from build123d import *

# Parameters (mm, degrees)
SKETCH1_W           = 30
SKETCH1_H           = 50
BOSS_EXTRUDE1_DEPTH = 10
SHELL1_T            = -3
CUT_EXTRUDE1_REACH  = 32.822
SKETCH2_R           = 1.5
SKETCH2_R_2         = 2.75
CUT_EXTRUDE2_REACH  = 42.311
SKETCH3_W           = 20
SKETCH3_H           = 5
FILLET1_R           = 2
FILLET2_R           = 2


with BuildPart() as part:
    # Sketch1 → Boss-Extrude1 (new body)
    with BuildSketch(Plane(origin=(0, 0, 0), x_dir=(1, 0, 0), z_dir=(0, 1, 0))):
        Rectangle(SKETCH1_W, SKETCH1_H)
    extrude(amount=BOSS_EXTRUDE1_DEPTH)

    # Shell1
    shell1_openings = [part.faces().sort_by_distance(p)[0] for p in [
        (0, 0, 0),
    ]]
    offset(amount=SHELL1_T, openings=shell1_openings, kind=Kind.INTERSECTION)

    # Sketch2 → Cut-Extrude1 (cut, up to next)
    with BuildSketch(Plane(origin=(0, 10, 0), x_dir=(1, 0, 0), z_dir=(0, 1, 0)), mode=Mode.PRIVATE) as cut_extrude1_sk1:
        with Locations(Location((0, -7, 0), (0, 0, 270))):
            Circle(SKETCH2_R)
    cut_extrude1_tool1 = extrude(cut_extrude1_sk1.sketch, amount=-CUT_EXTRUDE1_REACH, mode=Mode.PRIVATE) & part.part
    # Sketch2 → Cut-Extrude1 (cut, up to next)
    with BuildSketch(Plane(origin=(0, 10, 0), x_dir=(1, 0, 0), z_dir=(0, 1, 0)), mode=Mode.PRIVATE) as cut_extrude1_sk2:
        with Locations(Location((0, 5, 0), (0, 0, 270))):
            Circle(SKETCH2_R_2)
    cut_extrude1_tool2 = extrude(cut_extrude1_sk2.sketch, amount=-CUT_EXTRUDE1_REACH, mode=Mode.PRIVATE) & part.part
    add(cut_extrude1_tool1.solids().sort_by_distance((0, 10, 7))[0], mode=Mode.SUBTRACT)
    add(cut_extrude1_tool2.solids().sort_by_distance((0, 10, -5))[0], mode=Mode.SUBTRACT)

    # Sketch3 → Cut-Extrude2 (cut, up to next)
    with BuildSketch(Plane.ZY.offset(15), mode=Mode.PRIVATE) as cut_extrude2_sk1:
        with Locations((0, 2.5)):
            Rectangle(SKETCH3_W, SKETCH3_H)
    cut_extrude2_tool1 = extrude(cut_extrude2_sk1.sketch, amount=-CUT_EXTRUDE2_REACH, mode=Mode.PRIVATE) & part.part
    add(cut_extrude2_tool1.solids().sort_by_distance((-15, 2.5, 0))[0], mode=Mode.SUBTRACT)

    # Fillet1
    fillet1_edges = [part.edges().sort_by_distance(p)[0] for p in [
        (-13.5, 5, -10),
        (-13.5, 0, -10),
        (-13.5, 0, 10),
        (-13.5, 5, 10),
    ]]
    fillet(fillet1_edges, radius=FILLET1_R)

    # Fillet2
    fillet2_edges = [part.edges().sort_by_distance(p)[0] for p in [
        (-15, 10, 0),
        (0, 10, 25),
        (15, 10, 0),
        (0, 10, -25),
    ]]
    fillet(fillet2_edges, radius=FILLET2_R)


solid = part.part
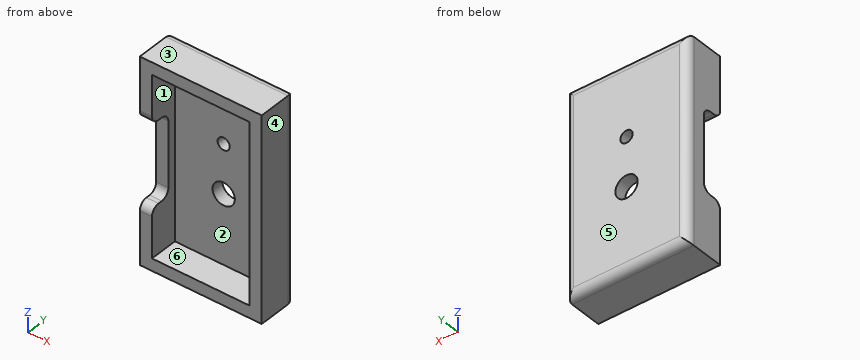
Verification items for the finished model (mm, model axes). Face numbers are marked on the shaded views. A direction names the side the tool comes from. Give positions to 0.01 mm unless a question says otherwise; leave off trailing zeros. Write each loop counter-clockwise with the first axis right and the second up, starting at its lowest first coordinate (ties: lowest second). Pieces come first, ordered by that corner, then holes. Notation, with made-up numbers: M 44.5,-40 L 80.5,-40 A36 ccw 80.5,-3 Z; hole C -19.5,86 d11. An arc over 180 degrees is marked long. Use CSV: the item, a comma, the result in double quotes.
1) Release check for a two-part mould opening along Z. For the marked faces 1, 2, 3 and 4 record: released by +Z, released by -Z, zero draft, split by the parting line, or undercut.
Final values:
face 1,"undercut"
face 2,"undercut"
face 3,"released by +Z"
face 4,"zero draft"
2) Cross-section at A-A (x = 0). Enter the section's corners in (y, z).
Final values:
outline,"M 0,-25 L 8,-25 A2 ccw 10,-23 L 10,-7.75 L 7,-7.75 L 7,-22 L 0,-22 Z; M 0,22 L 7,22 L 7,8.5 L 10,8.5 L 10,23 A2 ccw 8,25 L 0,25 Z; M 7,-2.25 L 10,-2.25 L 10,5.5 L 7,5.5 Z"
3) Go/stop test with flat-tipped pins: pin 1 Ø9 at (x, z) = (0, -5) entering from -Y; pin 2 Ø1.8 at (x, z) = (0, 7) entering from -Y; pin 3 Ø3.5 at (y, z) = (2, -5) entering from -X; pin 4 Ø1.5 at (x, z) = (-13.5, -1.5) entering from -Y. Record where each tip stops, or that it passes through.
Final values:
pin 1,"y = 7"
pin 2,"through"
pin 3,"x = 12"
pin 4,"y = 5"
4) Material ranges on line 1 along X through (y, z) = (1.5, 20); line 2 along Z through (x, y) = (-2.25, 5.75); line 3 along Y through (x, z) = (-13, 0.5), recorded low to high.
Final values:
line 1,"-15 to -12, 12 to 15"
line 2,"-25 to -22, 22 to 25"
line 3,"5 to 10"
5) Cross-section at D-D (x = -4.5). Enter the section's corners in (y, z), plus the area to 3 significant figures.
Final values:
outline,"M 0,-25 L 8,-25 A2 ccw 10,-23 L 10,23 A2 ccw 8,25 L 0,25 L 0,22 L 7,22 L 7,-22 L 0,-22 Z"
area,"190 mm²"
6) Cross-section at B-B (z = -5). Enter the section's corners in (x, y), plus the area to 3 significant figures.
Final values:
outline,"M -15,5 L -12,5 L -12,7 L -2.75,7 L -2.75,10 L -13,10 A2 ccw -15,8 Z; M 2.75,7 L 12,7 L 12,0 L 15,0 L 15,8 A2 ccw 13,10 L 2.75,10 Z"
area,"98.8 mm²"
7) Cross-section at C-C (z = 2). Enter the section's corners in (x, y).
Final values:
outline,"M -15,5 L -12,5 L -12,7 L 12,7 L 12,0 L 15,0 L 15,8 A2 ccw 13,10 L -13,10 A2 ccw -15,8 Z"
8) Access from +Z, -Z, +X, -X, +Y, -Y to the whole of each face (thin tool, end or side, straight path). Record for the marked faces 5 and 6.
Final values:
face 5,"+Z, -Z, +X, -X, +Y"
face 6,"-Y"
